Check sheet for the drawn part. Datum: minimum x, y, z corner. Units: mm. Give positions to 0.01 mm unless a question says otherwise; leave off trailing zeros. Order: outer loops, then holes, each group sorted by start corner. A loop starts at its lowest first (then second) coordinate and runs counter-clockwise, first axis right, second up. Notation, with made-up numbers: (18, -18) -> (52, -18) arc R25 ccw to (52, -2) -> close; hole circle Ø7 at (41, 85.25). An arc over 180 degrees is marked (long way). One line per question, with ' | ' between items. Start each with the question number.
Q1. Section check A-A on x = 7.5. Record the cut outline in (y, z).
Q2. Section check B-B on z = 4.5. Record the cut outline in (x, y).
Q3. Section check C-C on x = 13.5. Record the cut outline in (y, z).
Q4. Mould release check, pull along Z, two halves, no side actions. Record for the marked faces 1, 2 and 3: released by +Z, released by -Z, zero draft, split by the parting line, or undercut.
Q5. Go/stop test with flat-tipped pins: pin 1 (15 mm diameter, centred on x = 11.5, z = 28.5, fed in from +Y); pin 2 (4 mm diameter, centred on y = 4.5, z = 4, fed in from +X); pin 3 (1.9 mm diameter, centred on x = 24, y = 3.5, fed in from +Z); pin 4 (2 mm diameter, centred on x = 16, y = 1, fed in from -Z). Record where each tip stops, or that it passes through.
Q6. Material ranges on probe 1 along Y at (x, z) = (25.25, 19); probe 2 along Y at (x, z) = (4.5, 4); probe 3 along Z at (x, y) = (3.5, 2.75) (1 decimal), recorded low to high. Write a range as [from, to].
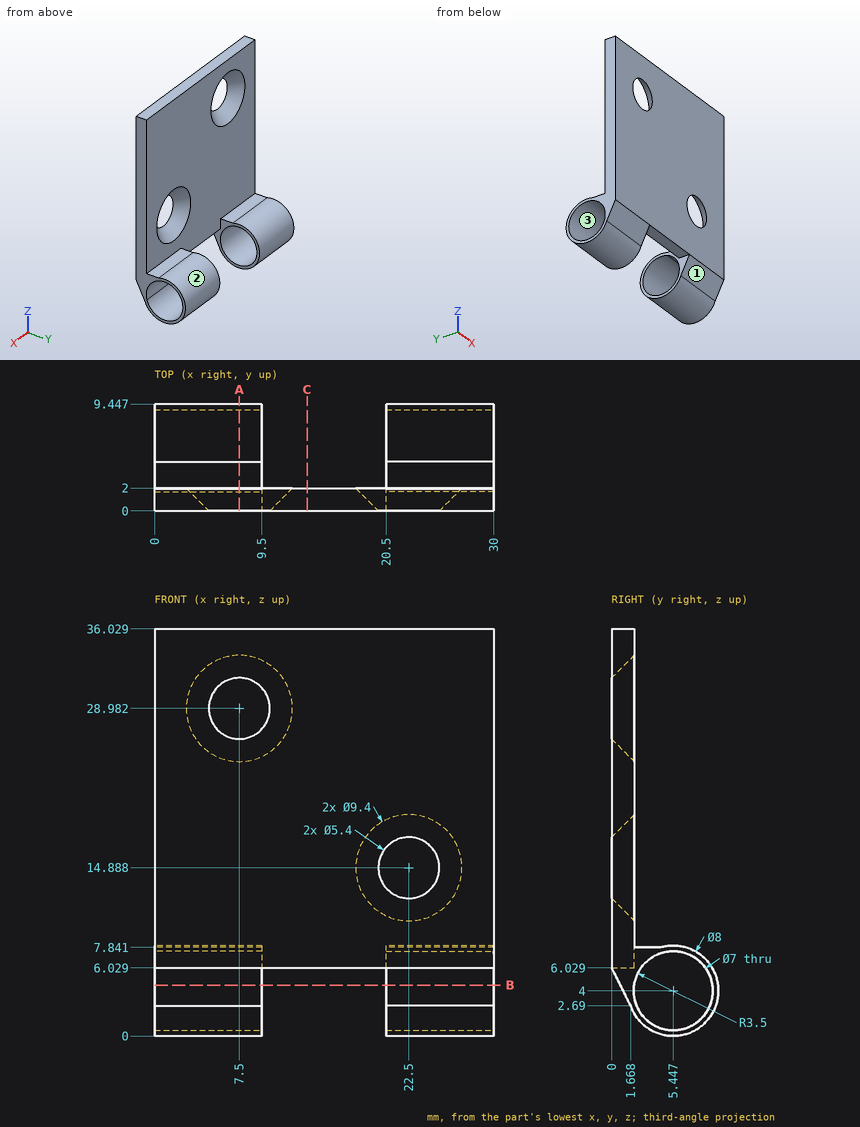
Filled in:
1) outline: (0, 6.03) -> (1.67, 2.69) arc R4 ccw (long way) to (4.33, 7.84) -> (2, 7.84) -> (2, 24.28) -> (0, 26.28) -> close; (0, 31.68) -> (2, 33.68) -> (2, 36.03) -> (0, 36.03) -> close; hole circle Ø7 at (5.45, 4)
2) outline: (0, 0.76) -> (9.5, 0.76) -> (9.5, 1.98) -> (0, 1.98) -> close; (0, 8.91) -> (9.5, 8.91) -> (9.5, 9.42) -> (0, 9.42) -> close; (20.5, 0.76) -> (30, 0.76) -> (30, 1.98) -> (20.5, 1.98) -> close; (20.5, 8.91) -> (30, 8.91) -> (30, 9.42) -> (20.5, 9.42) -> close
3) outline: (0, 6.03) -> (2, 6.03) -> (2, 36.03) -> (0, 36.03) -> close
4) face 1: released by -Z | face 2: split by the parting line | face 3: undercut
5) pin 1: y = 2 | pin 2: through | pin 3: z = 7.87 | pin 4: z = 6.03
6) probe 1: [0, 2] | probe 2: [1.01, 1.95], [8.95, 9.45] | probe 3: [1, 1.8], [6.2, 7.8]
